Drawing for the job (mm, zero at the part's lowest x, y, z). A direction names the side the tool comes from. Give positions to 0.01 mm unless a question says otherwise; leave off trailing zeros. Order: outer loops, then holes, each group sorted by start corner. A loop starts at its lowest first (then second) coordinate and runs counter-clockwise, first axis right, second up. Notation, with made-up numbers: (-6, 17.25) -> (36, 17.25) arc R27 cw to (36, 38.25) -> close; hole circle Ø2 at (88, 32). An arc over 180 degrees is marked (long way). Use a Markdown table: item, result. Add a question column.
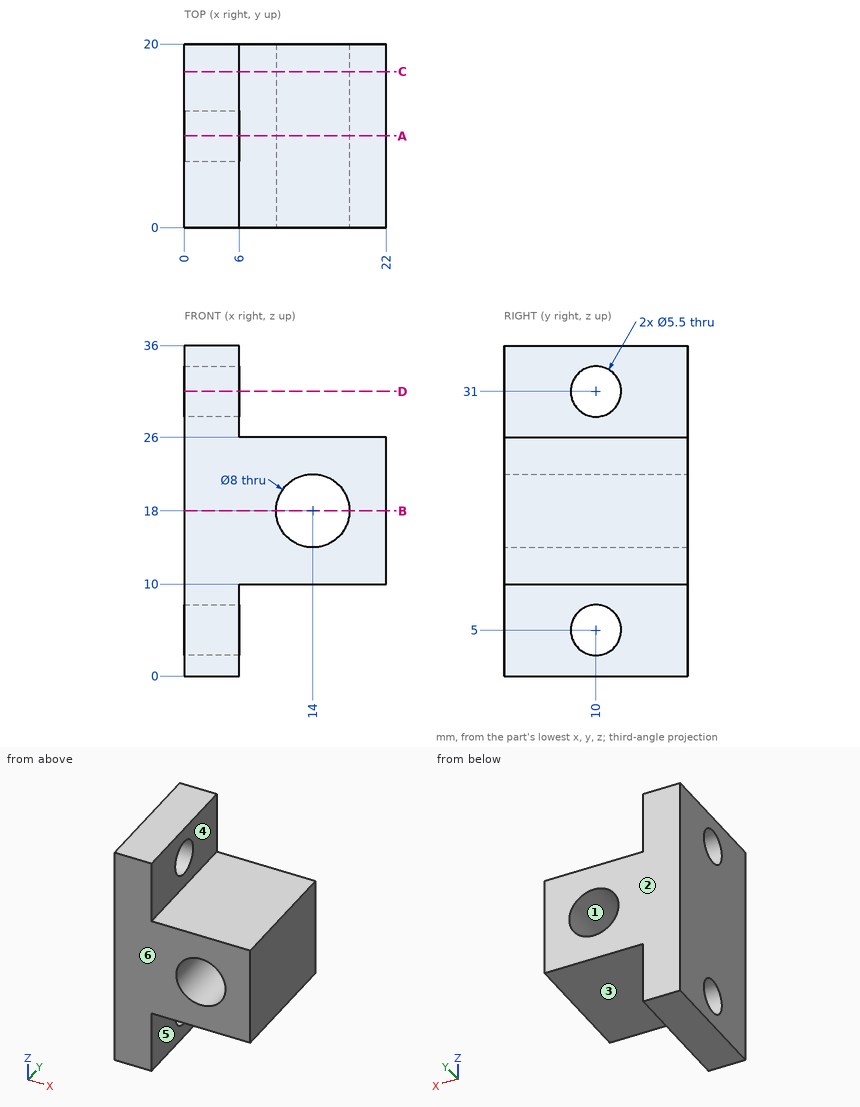
(1) Wall check: probe 1 along Y at (x, z) = (4.2, 5); probe 2 along Z at (x, y) = (7.25, 7.25); probe 3 along X at (y, z) = (5, 18). Give the ranges that are in metal, low to high.
(2) Band-saw the part on C-C on y = 17. Give the cut face in (x, z), plus the area to 3 significant figures.
(3) Band-saw the part on B-B on z = 18. Give the cut face in (x, y).
(4) Pin check, flat tips, straight feed: pin 1 Ø4 at (y, z) = (13, 6.5) entering from +X; pin 2 Ø2 at (x, y) = (16, 3.5) entering from -Z. Stop position of each tip, or through.
(5) Band-saw the part on A-A on y = 10. Give the cut face in (x, z).
(6) Tool access for the marked faces 4, 5 and 6: list every direction of +Z, -Z, +X, -X, +Y, -Y with a clear straight run to the whole face (end or side of a thin tool).
(7) Mould opens along Z. For the marked faces 1, 2 and 3 say: released by +Z, released by -Z, zero draft, split by the parting line, or undercut.
(8) Band-saw the part on D-D on z = 31. Give the cut face in (x, y), plus the area to 3 significant figures.
Response:
| question | item | result |
|---|---|---|
| 1 | probe 1 | y = 0 to 7.25, 12.75 to 20 |
| 1 | probe 2 | z = 10 to 26 |
| 1 | probe 3 | x = 0 to 10, 18 to 22 |
| 2 | outline | (0, 0) -> (6, 0) -> (6, 10) -> (22, 10) -> (22, 26) -> (6, 26) -> (6, 36) -> (0, 36) -> close; hole circle Ø8 at (14, 18) |
| 2 | area | 422 mm² |
| 3 | outline | (0, 0) -> (10, 0) -> (10, 20) -> (0, 20) -> close; (18, 0) -> (22, 0) -> (22, 20) -> (18, 20) -> close |
| 4 | pin 1 | stops at x = 6 |
| 4 | pin 2 | stops at z = 10 |
| 5 | outline | (0, 0) -> (6, 0) -> (6, 2.25) -> (0, 2.25) -> close; (0, 7.75) -> (6, 7.75) -> (6, 10) -> (22, 10) -> (22, 26) -> (6, 26) -> (6, 28.25) -> (0, 28.25) -> close; (0, 33.75) -> (6, 33.75) -> (6, 36) -> (0, 36) -> close; hole circle Ø8 at (14, 18) |
| 6 | face 4 | +Z, +X, +Y, -Y |
| 6 | face 5 | -Z, +X, +Y, -Y |
| 6 | face 6 | +Z, -Z, +X, -X, -Y |
| 7 | face 1 | undercut |
| 7 | face 2 | zero draft |
| 7 | face 3 | released by -Z |
| 8 | outline | (0, 0) -> (6, 0) -> (6, 7.25) -> (0, 7.25) -> close; (0, 12.75) -> (6, 12.75) -> (6, 20) -> (0, 20) -> close |
| 8 | area | 87.0 mm² |
